The drawing under review shows one solid part. Ordinate dimensions are in mm from its lowest x, y, z. A direction names the side the tool comes from. Coordinates: 2 decimals unless noted, no trailing zeros. Order: outer loops, then holes, each group sorted by start corner. A loop starts at its lowest first (then second) coordinate and runs counter-clockwise, first axis right, second up.
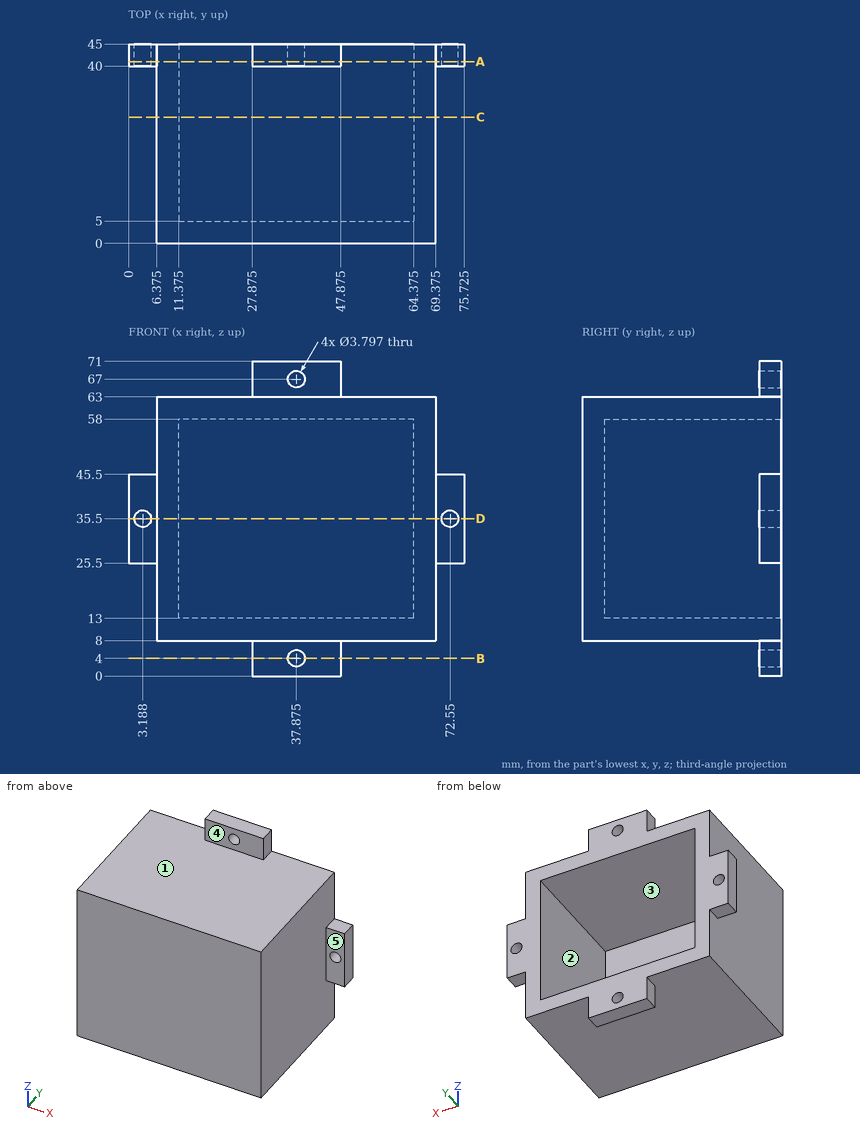
1. Machinability: for the marked faces 3, 4 and 5, which of the approach directions +Z, -Z, +X, -X, +Y, -Y give a long, thin tool a straight path to every point of the face, cutting with its end or side? Answer none if there is none.
Answer below:
face 3: +Y
face 4: +Z, +X, -X, -Y
face 5: +Z, -Z, +X, -Y
2. To check wall thickness, follow L1, parallel to X at y = 43.55, z = 35.5 (1 decimal); L2, parallel to Z at x = 16.5, y = 20.5; L3, parallel to X at y = 35, z = 28 (1 decimal). State the ranges of each line that lie inside material, in increasing order.
Answer below:
L1: x = 0 to 1.3, 5.1 to 11.4, 64.4 to 70.7, 74.4 to 75.7
L2: z = 8 to 13, 58 to 63
L3: x = 6.4 to 11.4, 64.4 to 69.4
3. Clearance check with flat-ended pins moving along their axes: pin 1 Ø5.5 at (y, z) = (42, 65.5) entering from +X (1 decimal); pin 2 Ø5 at (x, z) = (2, 38) entering from -Y; pin 3 Ø1.5 at (x, y) = (50, 30) entering from -Z; pin 4 Ø6 at (y, z) = (40, 25) entering from -X. State where each tip first meets the part, or that it passes through.
Answer below:
pin 1: stops at x = 69.4
pin 2: stops at y = 40
pin 3: stops at z = 8
pin 4: stops at x = 0
4. The part is to be moulded in two halves that separate along X. For the marked faces 1 and 2, say which applies: +X half, -X half, draft (parallel to the pull), parting line (faces both ways), or undercut.
Answer below:
face 1: draft
face 2: undercut
5. Take a section at D-D, the plane z = 35.5. Give the boundary of the cut face in (x, y) (1 decimal).
Answer below:
outline: (0, 40) - (1.3, 40) - (1.3, 45) - (0, 45) - close; (5.1, 40) - (6.4, 40) - (6.4, 0) - (69.4, 0) - (69.4, 40) - (70.7, 40) - (70.7, 45) - (64.4, 45) - (64.4, 5) - (11.4, 5) - (11.4, 45) - (5.1, 45) - close; (74.4, 40) - (75.7, 40) - (75.7, 45) - (74.4, 45) - close
6. Take a section at A-A, the plane y = 41. Give the number of separate pieces and of enclosed holes in the cut face, plus the area to 3 significant figures.
Answer below:
separate pieces: 1
enclosed holes: 5
area: 1,610 mm2
7. Take a section at B-B, the plane z = 4. Give the boundary of the cut face in (x, y) (1 decimal).
Answer below:
outline: (27.9, 40) - (36, 40) - (36, 45) - (27.9, 45) - close; (39.8, 40) - (47.9, 40) - (47.9, 45) - (39.8, 45) - close
8. Take a section at C-C, the plane y = 28.5. Give the boundary of the cut face in (x, z) (1 decimal).
Answer below:
outline: (6.4, 8) - (69.4, 8) - (69.4, 63) - (6.4, 63) - close; hole (11.4, 13) - (64.4, 13) - (64.4, 58) - (11.4, 58) - close
